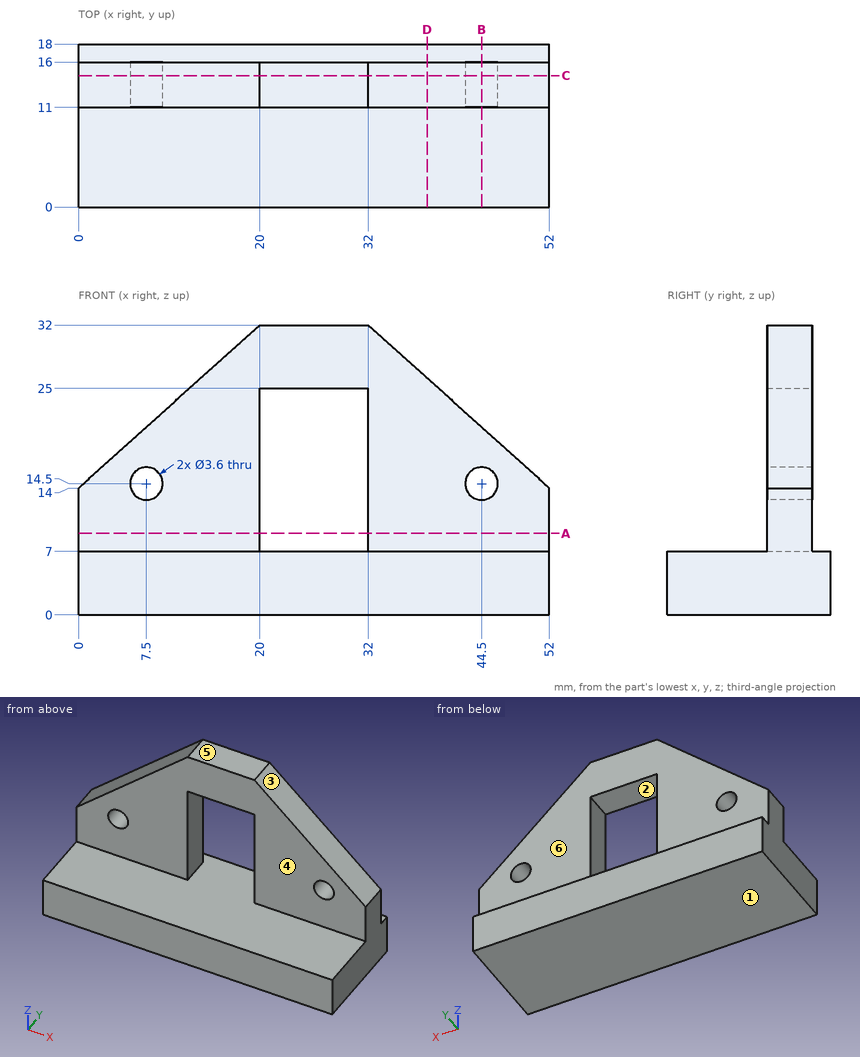
Geometry: see drawing. Coordinates: mm, zero at the bounding-box minimum. A direction names the side the tool comes from. Give positions to 0.01 mm unless a question says otherwise; leave off trailing zeros. Loops run counter-clockwise (first coordinate to the right, second up) from the corner with the lowest first, then second, coordinate; pieces in that order, holes last. Notation, with made-up numbers: (57, 20.25) -> (89, 20.25) arc R24 cw to (89, 30.25) -> close; hole circle Ø8 at (4, 44.25). An arc over 180 degrees is marked (long way). Answer as a JSON object with one key per item and string values. Group by question number.
Item 1: Pull-direction query (Z, two-part tool) for the marked faces 1, 2 and 3; classes: released by +Z, released by -Z, zero draft, split by the parting line, or undercut.
Item 2: Cut plane D-D, the plane x = 38.5. Return the cut outline in (y, z), and give its area (3 significant figures).
Item 3: Pin query (flat end, axial travel): P1, Ø1.5, axis at x = 38, z = 12.5, coming from the -Y side; P2, Ø1.5, axis at x = 24.5, y = 14.5, coming from the -Z side; P3, Ø4, axis at x = 42.5, y = 8.5, coming from the +Z side; P4, Ø2, axis at x = 13, y = 13.5, coming from the +Z side. Return the tip coordinate at first contact, or that it passes through.
Item 4: Cut plane C-C, the plane y = 14.5. Return the cut outline in (x, z).
Item 5: Line query: probe 1 along Z at (x, y) = (7.5, 14.15); probe 2 along Z at (x, y) = (18, 3). Output: solid intervals per line, ascending.
Item 6: Cut plane A-A, the plane z = 9. Return the cut outline in (x, y).
Item 7: Reachability of the marked faces 4, 5 and 6 from +Z, -Z, +X, -X, +Y, -Y: full face, straight path, thin tool, end or side. Return the list, or none.
Item 8: Cut plane B-B, the plane x = 44.5. Return the cut outline in (y, z).
Checks:
{
 "1": {"face 1": "released by -Z", "face 2": "undercut", "face 3": "released by +Z"},
 "2": {"outline": "(0, 0) -> (18, 0) -> (18, 7) -> (16, 7) -> (16, 26.15) -> (11, 26.15) -> (11, 7) -> (0, 7) -> close", "area": "222 mm²"},
 "3": {"P1": "stops at y = 11", "P2": "stops at z = 0", "P3": "stops at z = 7", "P4": "stops at z = 26.6"},
 "4": {"outline": "(0, 0) -> (52, 0) -> (52, 14) -> (32, 32) -> (20, 32) -> (0, 14) -> close; hole circle Ø3.6 at (7.5, 14.5); hole (20, 7) -> (32, 7) -> (32, 25) -> (20, 25) -> close; hole circle Ø3.6 at (44.5, 14.5)"},
 "5": {"probe 1": "z = 0 to 12.7, 16.3 to 20.75", "probe 2": "z = 0 to 7"},
 "6": {"outline": "(0, 11) -> (20, 11) -> (20, 16) -> (0, 16) -> close; (32, 11) -> (52, 11) -> (52, 16) -> (32, 16) -> close"},
 "7": {"face 4": "+Z, +X, -X, -Y", "face 5": "+Z, +X, -X, +Y, -Y", "face 6": "+Z, +X, -X, +Y"},
 "8": {"outline": "(0, 0) -> (18, 0) -> (18, 7) -> (16, 7) -> (16, 12.7) -> (11, 12.7) -> (11, 7) -> (0, 7) -> close; (11, 16.3) -> (16, 16.3) -> (16, 20.75) -> (11, 20.75) -> close"}
}
